Build history of the part. All positions in model axes, mm. A direction names the side the tool comes from. Give positions to 0.01 mm unless a question says otherwise; leave off trailing zeros. Loops run counter-clockwise (first coordinate to the right, second up) from the corner with the lowest first, then second, coordinate; pieces in that order, holes last. Notation, with made-up numbers: M 69,36.25 L 102,36.25 A29 cw 102,61.25 Z; hole C 65,50.5 d7. An arc over 180 degrees is marked long. Put each result on its own line as item: value.
```python
from build123d import *

# Parameters (mm, degrees)
F0_W     = 64.227912575
F0_H     = 69.2516341805
F1_DEPTH = 37.5227332115
F2_R     = 20.2179019698
F3_DEPTH = 93.5621410608
F4_W     = 13.437692076
F4_H     = 9.3960277736
F5_DEPTH = 134.1055929661


with BuildPart() as f1:
    # F0 (on Top) → F1 (new body)
    with BuildSketch(Plane.XY):
        with Locations((-2.0325984806, -3.0785240233)):
            Rectangle(F0_W, F0_H)
    extrude(amount=F1_DEPTH)

    # F2 (on face) → F3 (cut)
    with BuildSketch(Plane.XY.offset(37.5227332115)):
        Circle(F2_R)
    extrude(amount=-F3_DEPTH, mode=Mode.SUBTRACT)

    # F4 (on face) → F5 (cut)
    with BuildSketch(Plane.XY.offset(37.5227332115)):
        with Locations((-18.2582512498, -25.6907660514)):
            Rectangle(F4_W, F4_H)
        with Locations((-31.6959433258, -25.6907660514)):
            Rectangle(F4_W, F4_H)
        with Locations((-18.2582512498, -16.2947382778)):
            Rectangle(F4_W, F4_H)
        Polygon((-11.5394052118, -11.596724391), (-11.5394052118, -20.9927521646), (-8.1456769597, -20.9927521646), (-8.1456769597, -2.2006966174), (-24.9770972878, -2.2006966174), (-24.9770972878, -11.596724391), align=None)
        with Locations((-31.6959433258, -16.2947382778)):
            Rectangle(F4_W, F4_H)
    extrude(amount=-F5_DEPTH, mode=Mode.SUBTRACT)


solid = f1.part
```
Q1. Mould opens along X. For faces 1 (the flat face through (-24.977, -7, 19)), 2 (the cylindrical face through (16.73, 11.35, 19.02)), 3 (the flat face through (-34.147, 10, 18)), 4 (the flat face through (-2, 31.547, 18)) say: pulls with the +X half, pulls with the -X half, needs draft (parallel to the pull), parting line crosses it, or undercut.
Here are the results:
face 1: undercut
face 2: undercut
face 3: pulls with the -X half
face 4: needs draft
Q2. Slice it at B-B (y = 0). List the corners of the cut face in (x, z), and give its area (3 significant figures).
Here are the results:
outline: M -34.15,0 L -20.22,0 L -20.22,37.52 L -34.15,37.52 Z; M 20.22,0 L 30.08,0 L 30.08,37.52 L 20.22,37.52 Z
area: 893 mm²
Q3. Slice it at C-C (z = 32.5). List the corners of the cut face in (x, y).
Here are the results:
outline: M -34.15,-37.7 L 30.08,-37.7 L 30.08,31.55 L -34.15,31.55 L -34.15,-11.6 L -24.98,-11.6 L -24.98,-2.2 L -20.1,-2.2 A20.22 cw long -8.15,-18.5 L -8.15,-20.99 L -11.54,-20.99 L -11.54,-30.39 L -34.15,-30.39 Z
Q4. Tool access for faces 5 (the flat face through (-23, -2.201, 19)), 6 (the flat face through (-2, -37.704, 18)), 7 (the flat face through (-23, -30.389, 19)): list every direction of +Z, -Z, +X, -X, +Y, -Y with a clear straight run to the whole face (end or side of a thin tool).
Here are the results:
face 5: +Z, -Z
face 6: +Z, -Z, +X, -X, -Y
face 7: +Z, -Z, -X
Q5. Probe line 1 (X direction, y = 0, z = 18); line 2 (Y direction, x = 0, z = 30.5); line 3 (Y direction, x = -30, z = 27). List the from-to ranges inside material, lowest first. Write a range as from..to.
Here are the results:
line 1: -34.15..-20.22, 20.22..30.08
line 2: -37.7..-20.22, 20.22..31.55
line 3: -37.7..-30.39, -11.6..31.55
Q6. Slice it at A-A (x = -23). List the corners of the cut face in (y, z).
Here are the results:
outline: M -37.7,0 L -30.39,0 L -30.39,37.52 L -37.7,37.52 Z; M -2.2,0 L 31.55,0 L 31.55,37.52 L -2.2,37.52 Z
Q7. Drop a flat-ended pin along its axis: pin 1 Ø1.2 at (y, z) = (-20.5, 16) entering from -X. Give the stop position or say it passes through.
Here are the results:
pin 1: x = -11.54
